from build123d import *

# Parameters (mm, degrees)
F0_R     = 25
F0_R_2   = 5.5
F1_DEPTH = 2


with BuildPart() as f1:
    # F0 (on Right) → F1 (new body)
    with BuildSketch(Plane.YZ):
        Circle(F0_R)
        with BuildLine():
            ThreePointArc((-20.710142, -5.774083), (-20.442251, -4.119402), (-19.009279, -3.24973))
            Line((-19.009279, -3.24973), (-9.590252, -2.18014))
            ThreePointArc((-9.590252, -2.18014), (-8.371676, -2.431246), (-7.537353, -3.354223))
            ThreePointArc((-7.537353, -3.354223), (-5.833631, -5.833631), (-3.354223, -7.537353))
            ThreePointArc((-3.354223, -7.537353), (-2.431246, -8.371676), (-2.18014, -9.590252))
            Line((-2.18014, -9.590252), (-3.24973, -19.009279))
            ThreePointArc((-3.24973, -19.009279), (-4.119402, -20.442251), (-5.774083, -20.710142))
            ThreePointArc((-5.774083, -20.710142), (-15.202796, -15.202796), (-20.710142, -5.774083))
        make_face(mode=Mode.SUBTRACT)
        with BuildLine():
            ThreePointArc((5.774083, -20.710142), (4.119402, -20.442251), (3.24973, -19.009279))
            Line((3.24973, -19.009279), (2.18014, -9.590252))
            ThreePointArc((2.18014, -9.590252), (2.431246, -8.371676), (3.354223, -7.537353))
            ThreePointArc((3.354223, -7.537353), (5.833631, -5.833631), (7.537353, -3.354223))
            ThreePointArc((7.537353, -3.354223), (8.371676, -2.431246), (9.590252, -2.18014))
            Line((9.590252, -2.18014), (19.009279, -3.24973))
            ThreePointArc((19.009279, -3.24973), (20.442251, -4.119402), (20.710142, -5.774083))
            ThreePointArc((20.710142, -5.774083), (15.202796, -15.202796), (5.774083, -20.710142))
        make_face(mode=Mode.SUBTRACT)
        with BuildLine():
            ThreePointArc((-20.710142, 5.774083), (-15.202796, 15.202796), (-5.774083, 20.710142))
            ThreePointArc((-5.774083, 20.710142), (-4.119402, 20.442251), (-3.24973, 19.009279))
            Line((-3.24973, 19.009279), (-2.18014, 9.590252))
            ThreePointArc((-2.18014, 9.590252), (-2.431246, 8.371676), (-3.354223, 7.537353))
            ThreePointArc((-3.354223, 7.537353), (-5.833631, 5.833631), (-7.537353, 3.354223))
            ThreePointArc((-7.537353, 3.354223), (-8.371676, 2.431246), (-9.590252, 2.18014))
            Line((-9.590252, 2.18014), (-19.009279, 3.24973))
            ThreePointArc((-19.009279, 3.24973), (-20.442251, 4.119402), (-20.710142, 5.774083))
        make_face(mode=Mode.SUBTRACT)
        Circle(F0_R_2, mode=Mode.SUBTRACT)
        with BuildLine():
            Line((2.18014, 9.590252), (3.24973, 19.009279))
            ThreePointArc((3.24973, 19.009279), (4.119402, 20.442251), (5.774083, 20.710142))
            ThreePointArc((5.774083, 20.710142), (15.202796, 15.202796), (20.710142, 5.774083))
            ThreePointArc((20.710142, 5.774083), (20.442251, 4.119402), (19.009279, 3.24973))
            Line((19.009279, 3.24973), (9.590252, 2.18014))
            ThreePointArc((9.590252, 2.18014), (8.371676, 2.431246), (7.537353, 3.354223))
            ThreePointArc((7.537353, 3.354223), (5.833631, 5.833631), (3.354223, 7.537353))
            ThreePointArc((3.354223, 7.537353), (2.431246, 8.371676), (2.18014, 9.590252))
        make_face(mode=Mode.SUBTRACT)
    extrude(amount=F1_DEPTH)


solid = f1.part
Part model, mm, in its own coordinate system. Coordinates: 2 decimals unless noted, no trailing zeros. Loops run counter-clockwise (first coordinate to the right, second up) from the corner with the lowest first, then second, coordinate; pieces in that order, holes last. Notation, with made-up numbers: (81, -2.75) - (88, -2.75) arc R21 cw to (88, 35.25) - close; hole circle Ø1 at (11, -20). An arc over 180 degrees is marked (long way). Write each question's results on one line, items separated by ' | '. Start each with the question number.
Q1. Slice it at D-D on x = 0.3. Give the number of separate pieces and of enclosed holes in the cut face, and give its area (3 significant figures).
Q2. Slice it at C-C on z = 12.5. Give the cut face in (x, y), and give its area (3 significant figures).
Q3. Drop a flat-ended pin along its axis: pin 1 Ø1 at (x, z) = (0.5, -9.5) entering from +Y. Give the stop position or say it passes through.
Q4. Probe line 1 along Z through (x, y) = (1.5, 0); line 2 along Y through (x, z) = (0.3, -3.5); line 3 along Z through (x, y) = (0.6, -5). List the from-to ranges inside material, lowest first.
Q5. Slice it at A-A on y = 0. Give the cut face in (x, z), and give its area (3 significant figures).
Q6. Two-plate mould, pull along Z, no slides. Class faces 1 (the cylindrical face through (0.99, 2.42, -8.39)), 2 (the flat face through (0, 5, -5)): +Z half, -Z half, draft (parallel to the pull), parting line (faces both ways), or undercut.
Answer:
1) separate pieces: 1 | enclosed holes: 5 | area: 936 mm2
2) outline: (0, -21.65) - (2, -21.65) - (2, -17.49) - (0, -17.49) - close; (0, -2.51) - (2, -2.51) - (2, 2.51) - (0, 2.51) - close; (0, 17.49) - (2, 17.49) - (2, 21.65) - (0, 21.65) - close | area: 26.7 mm2
3) pin 1: stops at y = 23.32
4) line 1: z = -25 to -5.5, 5.5 to 25 | line 2: y = -24.75 to -19.78, -7.47 to -4.24, 4.24 to 7.47, 19.78 to 24.75 | line 3: z = -24.49 to -20.77, -6.56 to -2.29, 2.29 to 6.56, 20.77 to 24.49
5) outline: (0, -25) - (2, -25) - (2, -5.5) - (0, -5.5) - close; (0, 5.5) - (2, 5.5) - (2, 25) - (0, 25) - close | area: 78.0 mm2
6) face 1: undercut | face 2: draft
